from build123d import *

# Parameters (mm, degrees)
F0_W     = 21
F0_H     = 22
F0_W_2   = 6
F0_H_2   = 0.8
F0_R     = 1.8
F1_DEPTH = 3
F2_DEPTH = 3.9
F3_W     = 7
F3_H     = 3.2
F4_DEPTH = 25


with BuildPart() as f1:
    # F0 (on Top) → F1 (new body)
    with BuildSketch(Plane.XY):
        Rectangle(F0_W, F0_H)
        with Locations((0, -10)):
            Rectangle(F0_W_2, F0_H_2, mode=Mode.SUBTRACT)
        with Locations((0, -8)):
            Rectangle(F0_W_2, F0_H_2, mode=Mode.SUBTRACT)
        with Locations((0, -6)):
            Rectangle(F0_W_2, F0_H_2, mode=Mode.SUBTRACT)
        with Locations((0, -4)):
            Rectangle(F0_W_2, F0_H_2, mode=Mode.SUBTRACT)
        with Locations((0, -2)):
            Rectangle(F0_W_2, F0_H_2, mode=Mode.SUBTRACT)
        with Locations((-7, 0)):
            Circle(F0_R, mode=Mode.SUBTRACT)
        Rectangle(F0_W_2, F0_H_2, mode=Mode.SUBTRACT)
        with Locations((0, 2)):
            Rectangle(F0_W_2, F0_H_2, mode=Mode.SUBTRACT)
        with Locations((0, 4)):
            Rectangle(F0_W_2, F0_H_2, mode=Mode.SUBTRACT)
        with Locations((7, 0)):
            Circle(F0_R, mode=Mode.SUBTRACT)
        with Locations((0, 6)):
            Rectangle(F0_W_2, F0_H_2, mode=Mode.SUBTRACT)
        with Locations((0, 8)):
            Rectangle(F0_W_2, F0_H_2, mode=Mode.SUBTRACT)
        with Locations((0, 10)):
            Rectangle(F0_W_2, F0_H_2, mode=Mode.SUBTRACT)
    extrude(amount=F1_DEPTH)

    # F0 (on Top) → F2 (join)
    with BuildSketch(Plane.XY):
        with Locations((0, 8)):
            Rectangle(F0_W_2, F0_H_2)
        with Locations((0, 6)):
            Rectangle(F0_W_2, F0_H_2)
        with Locations((0, 4)):
            Rectangle(F0_W_2, F0_H_2)
        with Locations((0, 2)):
            Rectangle(F0_W_2, F0_H_2)
        Rectangle(F0_W_2, F0_H_2)
        with Locations((0, -2)):
            Rectangle(F0_W_2, F0_H_2)
        with Locations((0, -4)):
            Rectangle(F0_W_2, F0_H_2)
        with Locations((0, -6)):
            Rectangle(F0_W_2, F0_H_2)
        with Locations((0, -8)):
            Rectangle(F0_W_2, F0_H_2)
        with Locations((0, 10)):
            Rectangle(F0_W_2, F0_H_2)
        with Locations((0, -10)):
            Rectangle(F0_W_2, F0_H_2)
    extrude(amount=F2_DEPTH)

    # F3 (on face) → F4 (cut)
    with BuildSketch(Plane(origin=(0, 0, 0), x_dir=(1, 0, 0), z_dir=(0, 0, -1))):
        Rectangle(F3_W, F3_H)
    extrude(amount=-F4_DEPTH, mode=Mode.SUBTRACT)


solid = f1.part
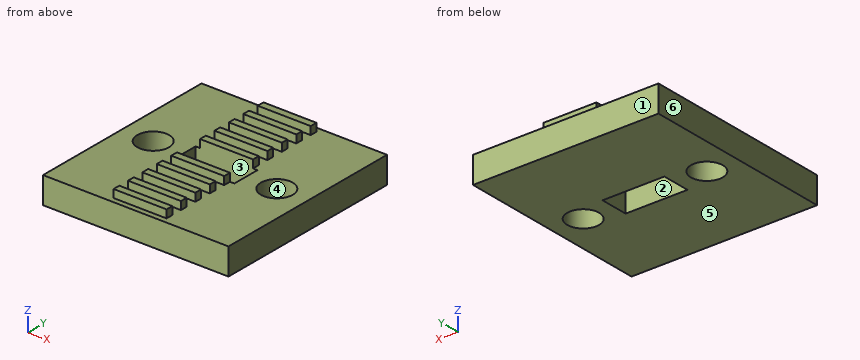
Input: part model. Units: mm. Frame: model coordinates. Face numbers are marked on the shaded views. A direction names the side the tool comes from. Coordinates: 2 decimals unless noted, no trailing zeros. Loops run counter-clockwise (first coordinate to the right, second up) from the corner with the lowest first, then second, coordinate; pieces in that order, holes last. Notation, with made-up numbers: (86.25, 29) - (92.25, 29) arc R30 ccw to (92.25, 68) - close; hole circle Ø2 at (19.25, 38.5). An arc over 180 degrees is marked (long way). Answer in a Markdown table with one row per item. Add a question column.
Item 1: Section query B-B on y = 0. Return the cut outline in (x, z), then the cut area to 3 significant figures.
Item 2: Mould query, pull axis X, two halves, no side actions, for the marked faces 3, 4, 5 and 6. Classes: released by +X, released by -X, zero draft, split by the parting line, or undercut.
Item 3: Section query A-A on x = 3.25. Return the cut outline in (y, z), then the cut area to 3 significant figures.
Item 4: Section query C-C on x = -7. Return the cut outline in (y, z), then the cut area to 3 significant figures.
Item 5: Section query D-D on z = 3.35. State how many separate pieces and enclosed holes the cut face has, then the cut area to 3 significant figures.
Item 6: Access query for the marked faces 1 and 2. Directions: +Z, -Z, +X, -X, +Y, -Y. A direction counts if a zero-diameter tool reaches every point of the face in a straight line with its end or side. Return the directions, or none.
Item 7: Line query: line 1 along Y through (x, z) = (2.5, 0.65); line 2 along Y through (x, z) = (-7, 1.3); line 3 along Z through (x, y) = (-3, 6.75). Output: solid intervals per line, ascending. Write a range as [from, to].
Item 8: Contact query for flat-ended pins moving along their axis: P1, Ø0.9, axis at y = -8, z = 3.5, coming from the +X side; P2, Ø0.9, axis at y = 4, z = 3.5, coming from the -X side; P3, Ø0.7, axis at x = 0, z = 3.5, coming from the -Y side. Output: stop coordinate, or through.
Recorded:
| question | item | result |
|---|---|---|
| 1 | outline | (-10.5, 0) - (-8.8, 0) - (-8.8, 3) - (-10.5, 3) - close; (-5.2, 0) - (-3.5, 0) - (-3.5, 3) - (-5.2, 3) - close; (3.5, 0) - (5.2, 0) - (5.2, 3) - (3.5, 3) - close; (8.8, 0) - (10.5, 0) - (10.5, 3) - (8.8, 3) - close |
| 1 | area | 20.4 mm^2 |
| 2 | face 3 | undercut |
| 2 | face 4 | undercut |
| 2 | face 5 | zero draft |
| 2 | face 6 | released by -X |
| 3 | outline | (-11, 0) - (-1.6, 0) - (-1.6, 3) - (-11, 3) - close; (1.6, 0) - (11, 0) - (11, 3) - (1.6, 3) - close |
| 3 | area | 56.4 mm^2 |
| 4 | outline | (-11, 0) - (-1.8, 0) - (-1.8, 3) - (-11, 3) - close; (1.8, 0) - (11, 0) - (11, 3) - (1.8, 3) - close |
| 4 | area | 55.2 mm^2 |
| 5 | separate pieces | 10 |
| 5 | enclosed holes | 0 |
| 5 | area | 48.0 mm^2 |
| 6 | face 1 | +Z, -Z, +X, -X, +Y |
| 6 | face 2 | +Z, -Z |
| 7 | line 1 | [-11, -1.6], [1.6, 11] |
| 7 | line 2 | [-11, -1.8], [1.8, 11] |
| 7 | line 3 | [0, 3] |
| 8 | P1 | x = 3 |
| 8 | P2 | x = -3 |
| 8 | P3 | y = -10.4 |
